```python
from build123d import *

# Parameters (mm, degrees)
SALIENTE_EXTRUIR1_DEPTH = 5
CROQUIS4_R              = 10
SALIENTE_EXTRUIR2_DEPTH = 10
CROQUIS5_R              = 1.5
SALIENTE_EXTRUIR3_DEPTH = 7
CORTAR_EXTRUIR1_REACH   = 110.601
CROQUIS6_W              = 6
CROQUIS6_H              = 4
CROQUIS7_W              = 5
CROQUIS7_H              = 5
CORTAR_EXTRUIR2_DEPTH   = 6


with BuildPart() as part:
    # Croquis2 → Recubrir1 section 0
    with BuildSketch(Plane(origin=(0, 40, 0), x_dir=(1, 0, 0), z_dir=(0, 1, 0))):
        with BuildLine():
            Line((15, -5), (-15, -5))
            Line((-15, -5), (-15, 5))
            Line((-15, 5), (15, 5))
            Line((15, 5), (15, -5))
        make_face()
    # Croquis1 → Recubrir1 section 1
    with BuildSketch(Plane(origin=(0, -40, 0), x_dir=(1, 0, 0), z_dir=(0, 1, 0))):
        with BuildLine():
            Line((-10, 10), (10, 10))
            Line((10, 10), (10, -10))
            Line((10, -10), (-10, -10))
            Line((-10, -10), (-10, 10))
        make_face()
    loft()

    # Croquis3 → Saliente-Extruir1 (add, symmetric)
    with BuildSketch(Plane(origin=(0, 0, 0), x_dir=(0, 0, -1), z_dir=(1, 0, 0))):
        with BuildLine():
            Line((-10, -40), (-11.882007165, -53.32133811))
            ThreePointArc((-11.882007165, -53.32133811), (0.627532313, -66.983580567), (11.641690846, -52.089495878))
            Line((11.641690846, -52.089495878), (10, -40))
            Line((10, -40), (-10, -40))
        make_face()
    extrude(amount=SALIENTE_EXTRUIR1_DEPTH, both=True)

    # Croquis4 → Saliente-Extruir2 (add, symmetric)
    with BuildSketch(Plane(origin=(0, 0, 0), x_dir=(0, 0, -1), z_dir=(1, 0, 0))):
        with Locations((0, -55)):
            Circle(CROQUIS4_R)
    extrude(amount=SALIENTE_EXTRUIR2_DEPTH, both=True)

    # Croquis5 → Saliente-Extruir3 (add)
    with BuildSketch(Plane(origin=(0, 0.46692607, 7.470817121), x_dir=(1, 0, 0), z_dir=(0, 0.062378286155180505, 0.9980525784828886))):
        with BuildLine():
            Line((6, 33.610211709), (-6, 33.610211709))
            ThreePointArc((-6, 33.610211709), (-9, 36.610211709), (-6, 39.610211709))
            Line((-6, 39.610211709), (6, 39.610211709))
            ThreePointArc((6, 39.610211709), (9, 36.610211709), (6, 33.610211709))
        make_face()
        with Locations(Location((-6, 36.610211709, 0), (0, 0, 270))):
            Circle(CROQUIS5_R, mode=Mode.SUBTRACT)
        with Locations(Location((6, 36.610211709, 0), (0, 0, 270))):
            Circle(CROQUIS5_R, mode=Mode.SUBTRACT)
    extrude(amount=SALIENTE_EXTRUIR3_DEPTH)

    # Cortar-Extruir1: up to this face of the body (flat: up to its plane)
    cortar_extruir1_end = Plane(part.part.faces().sort_by_distance((0, 34.230008531, 8.867453742))[0])
    # Croquis6 → Cortar-Extruir1 (cut, up to the picked face)
    with BuildSketch(Plane(origin=(0, 39.53307393, -2.470817121), x_dir=(1, 0, 0), z_dir=(0, 0.9980525784828886, -0.062378286155180505)), mode=Mode.PRIVATE) as cortar_extruir1_sk1:
        with Locations((6, -10.985394339)):
            Rectangle(CROQUIS6_W, CROQUIS6_H)
    cortar_extruir1_tool1 = split(extrude(cortar_extruir1_sk1.sketch, amount=-CORTAR_EXTRUIR1_REACH, mode=Mode.PRIVATE), bisect_by=cortar_extruir1_end, keep=Keep.BOTH, mode=Mode.PRIVATE)
    # Croquis6 → Cortar-Extruir1 (cut, up to the picked face)
    with BuildSketch(Plane(origin=(0, 39.53307393, -2.470817121), x_dir=(1, 0, 0), z_dir=(0, 0.9980525784828886, -0.062378286155180505)), mode=Mode.PRIVATE) as cortar_extruir1_sk2:
        with Locations((-6, -10.985394339)):
            Rectangle(CROQUIS6_W, CROQUIS6_H)
    cortar_extruir1_tool2 = split(extrude(cortar_extruir1_sk2.sketch, amount=-CORTAR_EXTRUIR1_REACH, mode=Mode.PRIVATE), bisect_by=cortar_extruir1_end, keep=Keep.BOTH, mode=Mode.PRIVATE)
    add(cortar_extruir1_tool1.solids().sort_by(Axis((6, 40.218324, 8.493184), (0, -0.9980525784828886, 0.062378286155180505)))[0], mode=Mode.SUBTRACT)
    add(cortar_extruir1_tool2.solids().sort_by(Axis((-6, 40.218324, 8.493184), (0, -0.9980525784828886, 0.062378286155180505)))[0], mode=Mode.SUBTRACT)

    # Croquis7 → Cortar-Extruir2 (cut)
    with BuildSketch(Plane(origin=(0, 39.53307393, -2.470817121), x_dir=(1, 0, 0), z_dir=(-1.2640787676290823e-15, 0.9980525784828886, -0.062378286155180505))):
        with Locations((0, -10.985394339)):
            Rectangle(CROQUIS7_W, CROQUIS7_H)
    extrude(amount=-CORTAR_EXTRUIR2_DEPTH, mode=Mode.SUBTRACT)


solid = part.part
```
Here's how the part is built. I have some questions about the finished solid (model axes, mm). A direction names the side the tool comes from. Coordinates: 2 decimals unless noted, no trailing zeros. Order: outer loops, then holes, each group sorted by start corner. A loop starts at its lowest first (then second) coordinate and runs counter-clockwise, first axis right, second up. Notation, with made-up numbers: (16, -31.75) - (65, -31.75) arc R16 ccw to (65, -25.75) - close; hole circle Ø5 at (28.5, 23). An arc over 180 degrees is marked (long way). One line per question, with ' | ' between items. Start each with the question number.
1. Please list where these lines run through material, in increasing order: line 1 along X through (y, z) = (-44.5, -3.5); line 2 along X through (y, z) = (-54, 9.5); line 3 along Y through (x, z) = (-8.5, 4.75). Write a range as [from, to].
2. If we mould it in two halves opening along Z, with no side actions, what happens to faces 4 (the flat face through (4.625, 36.06, 10.757)), 5 (the cylindrical face through (-9, 37, 6)), 6 (the flat face through (2.751, 34.227, 8.819)), 7 (the flat face through (5, -44, 0))? For each: released by +Z, released by -Z, zero draft, split by the parting line, or undercut.
3. If we section it at A-A (y = -55): Write out the boundary of the cut face in (x, z), and give its area (3 significant figures).
4. I'm going to push flat-ended pins straight in: pin 1 Ø5 at (x, z) = (-5.5, 4) entering from -Y; pin 2 Ø8 at (y, z) = (23, 6.5) entering from +X; pin 3 Ø8 at (y, z) = (19, 5.5) entering from -X. Where does each tip first touch, or does it pass through?
5. Which directions (+Z, -Z, +X, -X, +Y, -Y) give clear straight access to the entire face, cutting with the end or side of a thin tool? Please do faces 1 (the flat face through (10, -55, 0)), 2 (the flat face through (8, -40, 1)), 3 (the flat face through (-0.035, 37.422, 11.173)).
6. If we section it at B-B (z = 8): Give the number of separate pieces and of enclosed holes in the cut face, and give its area (3 significant figures).
Model answer:
1) line 1: x = [-5, 5] | line 2: x = [-10, 10] | line 3: y = [-63.8, -46.2], [-40, 40]
2) face 4: undercut | face 5: undercut | face 6: released by +Z | face 7: zero draft
3) outline: (-10, -10) - (-5, -10) - (-5, -12) - (5, -12) - (5, -10) - (10, -10) - (10, 10) - (5, 10) - (5, 12) - (-5, 12) - (-5, 10) - (-10, 10) - close | area: 440 mm²
4) pin 1: stops at y = -66.9 | pin 2: stops at x = 14.18 | pin 3: stops at x = -13.94
5) face 1: +Z, -Z, +X, -Y | face 2: +Z, -Z, +X | face 3: none
6) separate pieces: 3 | enclosed holes: 0 | area: 1,070 mm²
